from build123d import *

# Parameters (mm, degrees)
SKETCH1_W                = 69
SKETCH1_H                = 13.3
BOSS_EXTRUDE1_DEPTH      = 1.6
SKETCH2_W                = 69
SKETCH2_H                = 2
BOSS_EXTRUDE2_DEPTH      = 7.3
FILLET1_R                = 1
M2_START                 = -6.65
M2_CLEARANCE_SLOT1_DEPTH = 2


# Read off the part's stored shape, not the designer's step: M2 Clearance Slot1
with BuildPart() as part:
    # Sketch1 → Boss-Extrude1 (new body)
    with BuildSketch(Plane(origin=(0, 0, 0), x_dir=(1, 0, 0), z_dir=(0, 1, 0))):
        Rectangle(SKETCH1_W, SKETCH1_H)
    extrude(amount=BOSS_EXTRUDE1_DEPTH)

    # Sketch2 → Boss-Extrude2 (add)
    with BuildSketch(Plane(origin=(0, 1.6, 0), x_dir=(1, 0, 0), z_dir=(0, 1, 0))):
        with Locations((0, 5.65)):
            Rectangle(SKETCH2_W, SKETCH2_H)
    extrude(amount=BOSS_EXTRUDE2_DEPTH)

    # Fillet1
    fillet1_edges = [part.edges().sort_by_distance(p)[0] for p in [
        (0, 1.6, -4.65),
    ]]
    fillet(fillet1_edges, radius=FILLET1_R)

    # M2 Clearance Slot1 outline → M2 Clearance Slot1 (cut)
    with BuildSketch(Plane.XY.offset(M2_START)):
        with BuildLine():
            Line((23.2, 3.8), (23.2, 5.4))
            ThreePointArc((23.2, 5.4), (22, 6.6), (20.8, 5.4))
            Line((20.8, 5.4), (20.8, 3.8))
            ThreePointArc((20.8, 3.8), (22, 2.6), (23.2, 3.8))
        make_face()
        with BuildLine():
            Line((1.2, 3.8), (1.2, 5.4))
            ThreePointArc((1.2, 5.4), (0, 6.6), (-1.2, 5.4))
            Line((-1.2, 5.4), (-1.2, 3.8))
            ThreePointArc((-1.2, 3.8), (0, 2.6), (1.2, 3.8))
        make_face()
        with BuildLine():
            Line((-20.8, 3.8), (-20.8, 5.4))
            ThreePointArc((-20.8, 5.4), (-22, 6.6), (-23.2, 5.4))
            Line((-23.2, 5.4), (-23.2, 3.8))
            ThreePointArc((-23.2, 3.8), (-22, 2.6), (-20.8, 3.8))
        make_face()
    extrude(amount=M2_CLEARANCE_SLOT1_DEPTH, mode=Mode.SUBTRACT)


solid = part.part
Check sheet for the modelled part. Datum: model origin and axes. Units: mm. A direction names the side the tool comes from. Give positions to 0.01 mm unless a question says otherwise; leave off trailing zeros. Loops run counter-clockwise (first coordinate to the right, second up) from the corner with the lowest first, then second, coordinate; pieces in that order, holes last. Notation, with made-up numbers: M -26,22.25 L -1,22.25 A23 ccw -1,45.25 Z; hole C -34.5,4 d1. An arc over 180 degrees is marked long. Return JSON: item names as keys, results as strings. Group by question number.
1. Cross-section at B-B on z = 0.75. Record the boundary of the cut face in (x, y), plus the area to 3 significant figures.
2. Mould release check, pull along Y, two halves, no side actions. Record for faces 1 (the flat face through (0, 8.9, -6)), 2 (the flat face through (1.2, 5, -6)), 3 (the flat face through (0, 1, 6.65)): released by +Y, released by -Y, zero draft, split by the parting line, or undercut.
3. Thickness scan on L1, parallel to Z at x = 19, y = 6.5; L2, parallel to Y at x = -5, z = 0.5; L3, parallel to Y at x = -21.5, z = -5.25. Record the ranges inside material, lowest first.
4. Cross-section at A-A on x = -25. Record the boundary of the cut face in (y, z), plus the area to 3 significant figures.
5. Go/stop test with a flat-tipped pin: pin 1 (2 mm diameter, centred on x = -4, y = 6, fed in from +Z). Record where the tip stops, or that it passes through.
6. Tool access check on faces 4 (the cylindrical face through (-22, 6.6, -5.7)), 5 (the flat face through (34.5, 1, -2)), 6 (the flat face through (0, 1.6, 1)). Record the directions out of +Z, -Z, +X, -X, +Y, -Y that give a thin tool (end or side, any length) a straight path to the whole face; none if there is none.
Return value:
{
 "1": {"outline": "M -34.5,0 L 34.5,0 L 34.5,1.6 L -34.5,1.6 Z", "area": "110 mm^2"},
 "2": {"face 1": "released by +Y", "face 2": "undercut", "face 3": "zero draft"},
 "3": {"L1": "-6.65 to -4.65", "L2": "0 to 1.6", "L3": "0 to 2.71, 6.49 to 8.9"},
 "4": {"outline": "M 0,-6.65 L 8.9,-6.65 L 8.9,-4.65 L 2.6,-4.65 A1 cw 1.6,-3.65 L 1.6,6.65 L 0,6.65 Z", "area": "36.1 mm^2"},
 "5": {"pin 1": "z = -4.65"},
 "6": {"face 4": "+Z, -Z", "face 5": "+Z, -Z, +X, +Y, -Y", "face 6": "+Z, +X, -X, +Y"}
}
